from build123d import *

# Parameters (mm, degrees)
BOSS_EXTRUDE1_DEPTH = 1
SKETCH2_R           = 3
BOSS_EXTRUDE2_DEPTH = 3
CHAMFER1_SIZE       = 2
SKETCH3_R           = 1.5
CUT_EXTRUDE1_DEPTH  = 28.221315178
SKETCH4_R           = 1.5
CUT_EXTRUDE2_DEPTH  = 28.221315178


with BuildPart() as part:
    # Sketch1 → Boss-Extrude1 (new, symmetric)
    with BuildSketch(Plane.XY):
        with BuildLine():
            Line((-7, 0), (-4, 22))
            ThreePointArc((-4, 22), (0, 26), (4, 22))
            Line((4, 22), (7, 0))
            ThreePointArc((7, 0), (0, -7), (-7, 0))
        make_face()
    extrude(amount=BOSS_EXTRUDE1_DEPTH, both=True)

    # Sketch2 → Boss-Extrude2 (add, symmetric)
    with BuildSketch(Plane.XY):
        with BuildLine():
            Line((-5.909090909, 8), (5.909090909, 8))
            Line((5.909090909, 8), (7, 0))
            ThreePointArc((7, 0), (0, -7), (-7, 0))
            Line((-7, 0), (-5.909090909, 8))
        make_face()
        Circle(SKETCH2_R, mode=Mode.SUBTRACT)
    extrude(amount=BOSS_EXTRUDE2_DEPTH, both=True)

    # Chamfer1
    chamfer1_edges = [part.edges().sort_by_distance(p)[0] for p in [
        (0, 8, -3),
        (0, 8, 3),
    ]]
    chamfer(chamfer1_edges, length=CHAMFER1_SIZE - 0.0001)  # a hair under: the kernel refuses the full size

    # Sketch3 → Cut-Extrude1 (cut, through all)
    with BuildSketch(Plane.XY.offset(1)):
        with Locations((0, 22)):
            Circle(SKETCH3_R)
        with Locations((0, 17)):
            Circle(SKETCH3_R)
        with Locations((0, 12)):
            Circle(SKETCH3_R)
    extrude(amount=-CUT_EXTRUDE1_DEPTH, mode=Mode.SUBTRACT)

    # Sketch4 → Cut-Extrude2 (cut, through all)
    with BuildSketch(Plane.XY.offset(1)):
        Circle(SKETCH4_R)
    extrude(amount=-CUT_EXTRUDE2_DEPTH, mode=Mode.SUBTRACT)


solid = part.part
Read the model definition and answer for the solid it produces. Units are mm, in the model's axes. A direction names the side the tool comes from. Give positions to 0.01 mm unless a question says otherwise; leave off trailing zeros. Write each loop counter-clockwise with the first axis right and the second up, starting at its lowest first coordinate (ties: lowest second). Pieces come first, ordered by that corner, then holes. Notation, with made-up numbers: (75.25, -29.75) -> (131.25, -29.75) arc R8 cw to (131.25, -18.75) -> close; hole circle Ø6 at (-28, 67.5). An arc over 180 degrees is marked (long way). Answer as a JSON object with one key per item and string values. Group by question number.
1) Each of these flat-tipped pins is pushed along its axis until it touches: P1, Ø5, axis at x = 0, y = 22, coming from the +Z side; P2, Ø3, axis at x = -3, z = 2, coming from the +Y side; P3, Ø2, axis at x = -1.5, z = 1, coming from the +Y side. Where does it stop, or does it pass through?
2) The mould has two halves that part along Y. Classify faces 1 (the cylindrical face through (-3, 0, -2)), 2 (the flat face through (-3, 1, 3)), 3 (the cylindrical face through (0, -7, 0)): +Y half, -Y half, draft (parallel to the pull), parting line (faces both ways), or undercut.
3) A tool of negligible diameter and unlimited length cuts with its end or side. For faces 4 (the flat face through (-1.3, -1.3, -1)), 5 (the flat face through (-1.3, -1.3, 1)), 6 (the cylindrical face through (0, 26, 0)), 7 (the flat face through (0, 15, 1)), 8 (the flat face through (0, 15, -1)), from which of +Z, -Z, +X, -X, +Y, -Y can it reach the whole face along a straight path? Write none if from no direction.
4) Find section A-A (x = 0). Count the separate pieces of the cut face and the enclosed holes in it, and give its area (3 significant figures).
5) Consider L1, parallel to Y at x = 0, z = -0.2; L2, parallel to X at y = 0, z = 2; L3, parallel to Z at x = -0.5, y = 14. Determine where each line is inside the solid, lowest interval first. Write a range as from..to.
6) Find section B-B (y = 17). Write down the section's boundary in (x, z), and give its area (3 significant figures).
7) Find section D-D (z = -2.5). Write down the section's boundary in (x, y).
Values follow:
{
 "1": {"P1": "stops at z = 1", "P2": "stops at y = 25.53", "P3": "stops at y = 25.97"},
 "2": {"face 1": "undercut", "face 2": "draft", "face 3": "-Y half"},
 "3": {"face 4": "-Z", "face 5": "+Z", "face 6": "+Z, -Z, +Y", "face 7": "+Z, +X, -X, +Y", "face 8": "-Z, +X, -X, +Y"},
 "4": {"separate pieces": "5", "enclosed holes": "0", "area": "74.0 mm2"},
 "5": {"L1": "y = -7..-1.5, 1.5..10.5, 13.5..15.5, 18.5..20.5, 23.5..26", "L2": "x = -7..-3, 3..7", "L3": "z = -1..1"},
 "6": {"outline": "(-4.68, -1) -> (-1.5, -1) -> (-1.5, 1) -> (-4.68, 1) -> close; (1.5, -1) -> (4.68, -1) -> (4.68, 1) -> (1.5, 1) -> close", "area": "12.7 mm2"},
 "7": {"outline": "(-7, 0) arc R7 ccw to (7, 0) -> (6.11, 6.5) -> (-6.11, 6.5) -> close; hole circle Ø6 at (0, 0)"}
}
